```python
from build123d import *

# Parameters (mm, degrees)
F6_COPIES_COUNT = 4
F7_R            = 1


# Not quite as in the source:
# - a pattern or mirror of a feature is missing from the dataset's text; its kind, count and spacing are read off the source's solid


with BuildPart() as f4:
    # F3 (on Front) → F4 (revolve)
    with BuildSketch(Plane.XZ):
        Polygon((0, 0), (0, 8.46), (-15, 8.46), (-15, -3.54), (-13, -3.54), (-13, 0), align=None)
    revolve(axis=Axis((0, 0, -4.2355582118), (0, 0, -1)))

    # F5 (on Front) → F6 (revolve, cut)
    with BuildSketch(Plane.XZ):
        Polygon((-0.1761714047, -0.0391753335), (-5.0730880905, 3.4278416801), (-8.3376992144, 5.7391863558), (-7.5865121948, 6.800184971), (-14.1157344425, 11.4228743224), (-17.2938333716, 6.9340340271), (-7.5, 0), (-2.5972818806, -3.4588228983), align=None)
    f6 = revolve(axis=Axis((-9.8969166858, 0, 1.6970170136), (-0.816152781, 0, 0.5778361689)), mode=Mode.SUBTRACT)

    # F6_copies: F6 ×4 about axis
    f6_copies_axis = Axis((0, 0, 0), (0, 0, 1))
    for i in range(1, F6_COPIES_COUNT):
        add(f6.rotate(f6_copies_axis, i * 360 / F6_COPIES_COUNT), mode=Mode.SUBTRACT)

    # F7
    f7_edges = [f4.edges().sort_by_distance(p)[0] for p in [
        (-10.606602, 10.606602, 8.46),
        (10.606602, 10.606602, 8.46),
        (10.606602, -10.606602, 8.46),
        (-10.606602, -10.606602, 8.46),
    ]]
    fillet(f7_edges, radius=F7_R)


solid = f4.part
```
Model file for the job. Use its own axes, mm. A direction names the side the tool comes from. Coordinates: 2 decimals unless noted, no trailing zeros. Answer as a JSON object with one key per item and string values.
Q1. Flat gauge pins, fed straight in: P1, Ø7.5, axis at x = 7, y = 5.5, coming from the -Z side; P2, Ø1, axis at y = -7, z = 6.5, coming from the -X side; P3, Ø4, axis at x = 0.5, z = 4.5, coming from the -Y side. Where does each tip first touch, or does it go through?
Report:
{"P1": "stops at z = 0", "P2": "stops at x = -13.52", "P3": "stops at y = -8.77"}
Q2. 3-axis set-ups, long thin cutter, end or side, ignore diameter. For faces 1 (the flat face through (-7, -7, 0)), 2 (the cylindrical face through (5.243, 0.136, 3.546)): which of +Z, -Z, +X, -X, +Y, -Y reach the whole face in a straight line?
Report:
{"face 1": "-Z", "face 2": "none"}
Q3. Pull direction Y, two halves, no side cores. Call faces 3 (the cylindrical face through (-13.856, -5.745, 0.661)), 4 (the cylindrical face through (-1.652, -9.668, 7.963)), 5 (the flat face through (0.1, 13.4, -3.54)): released by +Y, released by -Y, zero draft, split by the parting line, or undercut.
Report:
{"face 3": "split by the parting line", "face 4": "undercut", "face 5": "zero draft"}
Q4. Cut at A-A (y = -1). State how many separate pieces and enclosed holes the cut face has, and give its area (3 significant figures).
Report:
{"separate pieces": "3", "enclosed holes": "0", "area": "105 mm2"}
Q5. Probe probe 1 along Y at (x, z) = (0, -2.35); probe 2 along Y at (x, z) = (0, -2.1). List the from-to ranges inside material, lowest first.
Report:
{"probe 1": "y = -15 to -13, 13 to 15", "probe 2": "y = -15 to -14.05, -13.89 to -13, 13 to 13.89, 14.05 to 15"}
